Verification items for the finished model (mm, model axes). A direction names the side the tool comes from. Give positions to 0.01 mm unless a question says otherwise; leave off trailing zeros. Loops run counter-clockwise (first coordinate to the right, second up) from the corner with the lowest first, then second, coordinate; pieces in that order, holes last. Notation, with made-up numbers: (-29.5, 60.5) - (27.5, 60.5) arc R23 cw to (27.5, 81.5) - close; hole circle Ø9 at (15.25, 5.25). An arc over 180 degrees is marked (long way). Use one line per item in the form item = value.
```python
from build123d import *

# Parameters (mm, degrees)
F0_W     = 152.4
F0_H     = 152.4
F1_DEPTH = 3.175
F3_DEPTH = 6.35


# Not quite as in the source:
# - a length typed as a fraction of an inch, garbled in the dataset ("3 / 203.2 mm" for 3/8 in), is restored
# - a feature names something its author has since deleted; it is built from what else it names


with BuildPart() as f1:
    # F0 (on Front) → F1 (new body)
    with BuildSketch(Plane.XZ):
        with Locations((9.2369243503, 5.9638554769)):
            Rectangle(F0_W, F0_H)
    extrude(amount=F1_DEPTH)

    # F2 (on Right) → F3 (join)
    with BuildSketch(Plane.YZ):
        Polygon((0, 0), (0, 49.6197640896), (-75.9790167212, 49.6197640896), (-75.9790167212, -51.2280538678), (0, -51.2280538678), align=None)
    extrude(amount=F3_DEPTH)


solid = f1.part
```
1. Scan lines: probe 1 along X at (y, z) = (-12, 34); probe 2 along Y at (x, z) = (32, 73.5) (3 decimals); probe 3 along Z at (x, y) = (4.5, -9). Record each from-to range of solid material in increasing order.
Result set:
probe_1 = 0 to 6.35
probe_2 = -3.175 to 0
probe_3 = -51.23 to 49.62
2. Depth check by flat-ended pin: pin 1 Ø7 at (x, y) = (4, -54) entering from -Z; pin 2 Ø4 at (y, z) = (-21, 48) entering from -X; pin 3 Ø7 at (x, y) = (3, -30) entering from +Z. Enter the tip coordinate at first touch or a pass-through.
Result set:
pin_1 = -51.23
pin_2 = 0
pin_3 = 49.62
3. Section check C-C, the plane x = -22. Record the cut outline in (y, z) (3 decimals).
Result set:
outline = (-3.175, -70.236) - (0, -70.236) - (0, 82.164) - (-3.175, 82.164) - close
4. Section check B-B, the plane y = -64. Record the cut outline in (x, z), then the cut area to 3 significant figures.
Result set:
outline = (0, -51.23) - (6.35, -51.23) - (6.35, 49.62) - (0, 49.62) - close
area = 640 mm²
5. Tool access check on faces 1 (the flat face through (6.35, -40, 0)), 2 (the flat face through (3, -40, -51.228)), 3 (the flat face through (3, -39, 49.62)), 4 (the flat face through (0, -40, 0)). Record the directions out of +Z, -Z, +X, -X, +Y, -Y that give a thin tool (end or side, any length) a straight path to the whole face; none if there is none.
Result set:
face_1 = +Z, -Z, +X, -Y
face_2 = -Z, +X, -X, -Y
face_3 = +Z, +X, -X, -Y
face_4 = +Z, -Z, -X, -Y
6. Section check A-A, the plane z = -28. Record the cut outline in (x, y) (3 decimals).
Result set:
outline = (-66.963, -3.175) - (0, -3.175) - (0, -75.979) - (6.35, -75.979) - (6.35, -3.175) - (85.437, -3.175) - (85.437, 0) - (-66.963, 0) - close
